For this review, take the finished solid that the model builds, in its own axes (mm). Face numbers are marked on the shaded views. A direction names the side the tool comes from. Coordinates: 2 decimals unless noted, no trailing zeros. Loops run counter-clockwise (first coordinate to the right, second up) from the corner with the lowest first, then second, coordinate; pieces in that order, holes last. Notation, with made-up numbers: (79, 35) - (130, 35) arc R9 cw to (130, 44) - close; hole circle Ø4 at (11, 29). An arc over 180 degrees is marked (long way). Answer as a JSON object with one key per item and string values. Group by question number.
Item 1: We need section B-B (x = -2.25). Give the boundary of the cut face in (y, z).
Item 2: Tool access review of the marked faces 5 and 6: name each direction out of +Z, -Z, +X, -X, +Y, -Y from which nothing blocks a thin tool from reaching the whole face with its end or side.
Item 3: Mouldability with a two-part tool opening along Y and no side actions: class the marked faces 1, 2, 3 and 4 as released by +Y, released by -Y, zero draft, split by the parting line, or undercut.
Item 4: Clearance check with flat-ended pins moving along their axes: pin 1 (0.9 mm diameter, centred on y = 1, z = -3, fed in from +X); pin 2 (0.9 mm diameter, centred on x = -1, y = 1.5, fed in from -Z); pin 3 (8.5 mm diameter, centred on y = -13, z = 4, fed in from -X); pin 4 (2 mm diameter, centred on y = 1.5, z = 6, fed in from -X). State where each tip first meets the part, or that it passes through.
Item 5: To check wall thickness, follow line 1 (Z direction, x = 1.75, y = -28); line 2 (Z direction, x = -4.5, y = -27); line 3 (X direction, y = -3.5, z = 0). State the ranges of each line that lie inside material, in increasing order.
Item 6: We need section A-A (y = -14.5). Give the boundary of the cut face in (x, z), then the cut area to 3 significant figures.
Item 7: We need section D-D (x = 4.5). Give the boundary of the cut face in (y, z).
Item 8: We need section C-C (y = -8). Give the boundary of the cut face in (x, z), then the cut area to 3 significant figures.
from build123d import *

# Parameters (mm, degrees)
SKETCH1_W           = 8
SKETCH1_H           = 27.5
BOSS_EXTRUDE1_DEPTH = 3
SKETCH2_W           = 10
SKETCH2_H           = 30
BOSS_EXTRUDE2_DEPTH = 10
SKETCH4_W           = 10
SKETCH4_H           = 5
BOSS_EXTRUDE3_DEPTH = 20
CHAMFER2_SIZE       = 5
CHAMFER2_SIZE2      = 15
SKETCH7_W           = 4
SKETCH7_H           = 5
CUT_EXTRUDE2_DEPTH  = 2
SHELL1_START        = -4
SHELL1_DEPTH        = 8
SHELL1_START_2      = -3
SHELL1_2_OUTLINE_W  = 4
SHELL1_2_OUTLINE_H  = 25.5
SHELL1_2_DEPTH      = 6
SHELL1_START_3      = -1
SHELL1_3_DEPTH      = 5


# Read off the part's stored shape, not the designer's step: Shell1
with BuildPart() as part:
    # Sketch1 → Boss-Extrude1 (new body)
    with BuildSketch(Plane(origin=(0, 0, 0), x_dir=(1, 0, 0), z_dir=(0, 1, 0))):
        Rectangle(SKETCH1_W, SKETCH1_H)
    extrude(amount=BOSS_EXTRUDE1_DEPTH)

    # Sketch2 → Boss-Extrude2 (add)
    with BuildSketch(Plane.XZ):
        Rectangle(SKETCH2_W, SKETCH2_H)
    extrude(amount=BOSS_EXTRUDE2_DEPTH)

    # Sketch4 → Boss-Extrude3 (add)
    with BuildSketch(Plane.XZ.offset(10)):
        with Locations((0, 12.5)):
            Rectangle(SKETCH4_W, SKETCH4_H)
        with Locations((0, -12.5)):
            Rectangle(SKETCH4_W, SKETCH4_H)
    extrude(amount=BOSS_EXTRUDE3_DEPTH)

    # Chamfer2
    chamfer2_edges = [part.edges().sort_by_distance(p)[0] for p in [
        (0, -10, 10),
        (0, -10, -10),
    ]]
    chamfer2_side = [part.faces().sort_by_distance(p)[0] for p in [
        (0, -10, 0),
    ]]
    chamfer(chamfer2_edges, length=CHAMFER2_SIZE, length2=CHAMFER2_SIZE2, reference=chamfer2_side[0])

    # Sketch7 → Cut-Extrude2 (cut)
    with BuildSketch(Plane(origin=(0, 0, 10), x_dir=(-1, 0, 0), z_dir=(0, 0, -1))):
        with Locations((3, -27.5)):
            Rectangle(SKETCH7_W, SKETCH7_H)
    extrude(amount=-CUT_EXTRUDE2_DEPTH, mode=Mode.SUBTRACT)

    # Shell1 outline → Shell1 (cut)
    with BuildSketch(Plane.YZ.offset(SHELL1_START)):
        Polygon((-9, 5.72075922), (-9, -5.72075922), (-24.83772234, -11), (-29, -11), (-29, -14), (-1, -14), (-1, 14), (-29, 14), (-29, 11), (-25, 11), (-25, 11.054092553), align=None)
    extrude(amount=SHELL1_DEPTH, mode=Mode.SUBTRACT)

    # Shell1 2 outline → Shell1 2 (cut)
    with BuildSketch(Plane.YZ.offset(SHELL1_START_2)):
        with Locations((1, 0)):
            Rectangle(SHELL1_2_OUTLINE_W, SHELL1_2_OUTLINE_H)
    extrude(amount=SHELL1_2_DEPTH, mode=Mode.SUBTRACT)

    # Shell1 3 outline → Shell1 3 (cut)
    with BuildSketch(Plane.YZ.offset(SHELL1_START_3)):
        Polygon((-25, 11), (-24.83772234, 11), (-25, 11.054092553), align=None)
    extrude(amount=SHELL1_3_DEPTH, mode=Mode.SUBTRACT)


solid = part.part
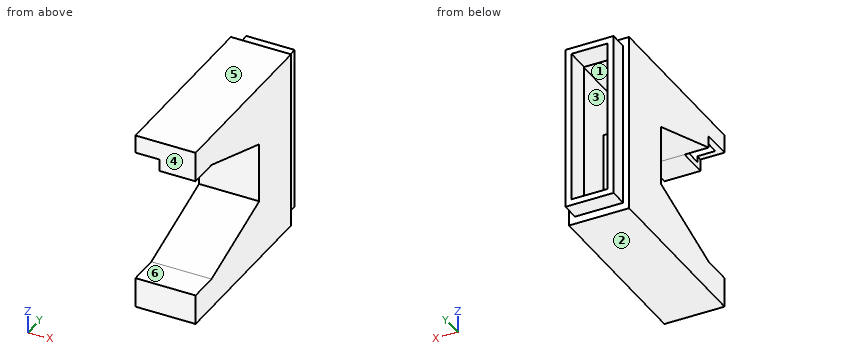
Check sheet entries:
{
 "1": {"outline": "(-30, -15) - (0, -15) - (0, -13.75) - (3, -13.75) - (3, -12.75) - (-1, -12.75) - (-1, -14) - (-29, -14) - (-29, -11) - (-24.84, -11) - (-9, -5.72) - (-9, 5.72) - (-25, 11.05) - (-25, 10) - (-10, 5) - (-10, -5) - (-25, -10) - (-30, -10) - close; (-30, 12) - (-29, 12) - (-29, 14) - (-1, 14) - (-1, 12.75) - (3, 12.75) - (3, 13.75) - (0, 13.75) - (0, 15) - (-30, 15) - close"},
 "2": {"face 5": "+Z, +X, -X, +Y, -Y", "face 6": "+X, -X, -Y"},
 "3": {"face 1": "undercut", "face 2": "zero draft", "face 3": "undercut", "face 4": "released by -Y"},
 "4": {"pin 1": "stops at x = 4", "pin 2": "stops at z = -13.75", "pin 3": "stops at x = -5", "pin 4": "stops at x = -4"},
 "5": {"line 1": "z = -15 to -14, -11 to -10, 10 to 11, 14 to 15", "line 2": "z = -15 to -10, 12 to 15", "line 3": "x = -5 to -4, 4 to 5"},
 "6": {"outline": "(-5, -15) - (5, -15) - (5, -6.5) - (-5, -6.5) - close; (-5, 6.5) - (5, 6.5) - (5, 15) - (-5, 15) - close; hole (-4, -14) - (4, -14) - (4, -7.55) - (-4, -7.55) - close; hole (-4, 7.55) - (4, 7.55) - (4, 14) - (-4, 14) - close", "area": "66.9 mm2"},
 "7": {"outline": "(-30, -15) - (0, -15) - (0, 15) - (-30, 15) - (-30, 10) - (-25, 10) - (-10, 5) - (-10, -5) - (-25, -10) - (-30, -10) - close"},
 "8": {"outline": "(-5, -15) - (5, -15) - (5, 15) - (-5, 15) - close; hole (-4, -14) - (4, -14) - (4, 14) - (-4, 14) - close", "area": "76.0 mm2"}
}
